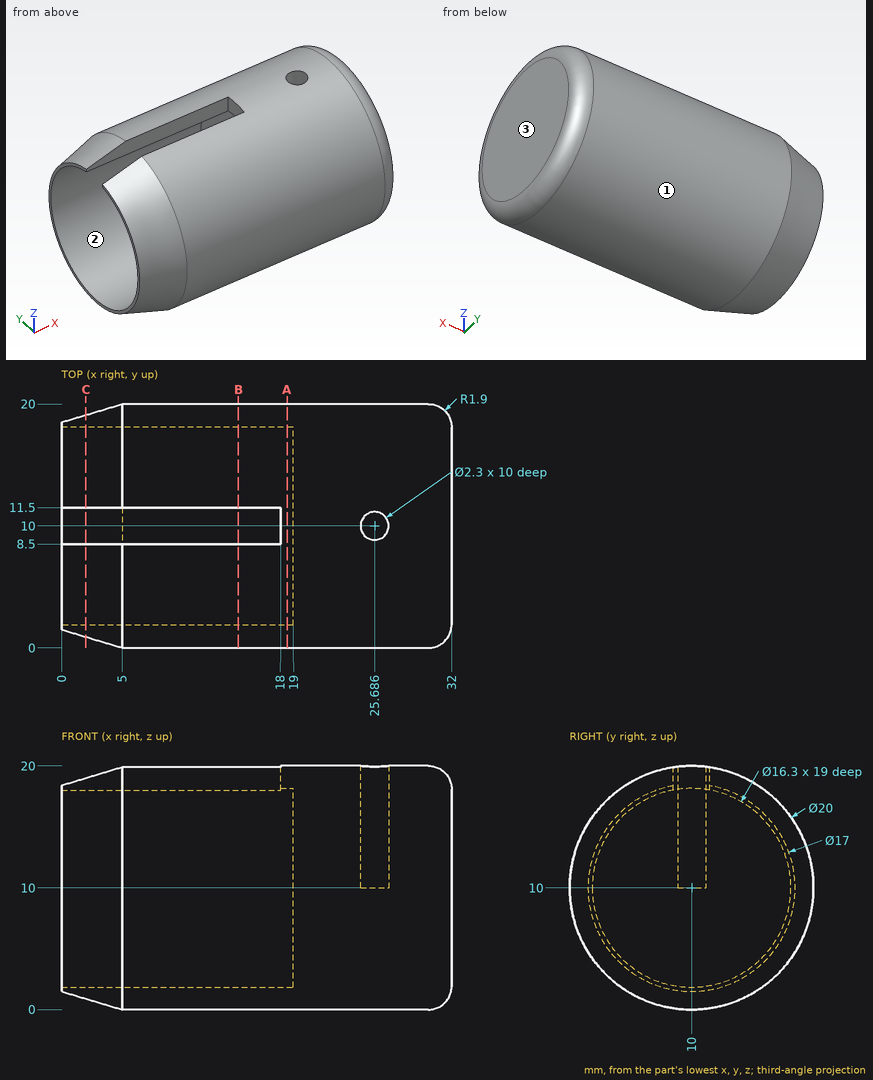
For this review, use the dimensioned drawing (mm, ordinates from the lowest corner) and the shaded views. Give positions to 0.01 mm unless a question says otherwise; leave off trailing zeros. Write each loop counter-clockwise with the first axis right and the second up, starting at its lowest first coordinate (ties: lowest second). Pieces come first, ordered by that corner, then holes.
(1) Consider section B-B, the plane x = 14.5. Give the boundary of the cut face in (y, z).
(2) For P1, Ø1, axis at x = 4.5, z = 16.5, coming from the -Y side; P2, Ø1, axis at x = 25, z = 3.5, coming from the -Y side; P3, Ø4, axis at x = 11, y = 16, coming from the -Z side, all flat-tipped, find the tip position at first contact; note any pin that passes through.
(3) Consider section C-C, the plane x = 2. Give the boundary of the cut face in (y, z), and give its area (3 significant figures).
(4) The part is to be moulded in two halves that separate along Y. For the marked faces 1, 2 and 3, say which applies: released by +Y, released by -Y, zero draft, split by the parting line, or undercut.
(5) To check wall thickness, follow L1, parallel to Y at x = 11, z = 14.75; L2, parallel to Y at x = 4.5, z = 2.5; L3, parallel to X at y = 11.5, z = 10.75. State the ranges of each line that lie inside material, in increasing order.
(6) Consider section A-A, the plane x = 18.5. Give the boundary of the cut face in (y, z).
Returned:
1. outline: (8.5, 18.01) - (8.5, 19.89) arc R10 ccw (long way) to (11.5, 19.89) - (11.5, 18.01) arc R8.15 cw (long way) to start
2. P1: stops at y = 2.14
2. P2: stops at y = 2
2. P3: stops at z = 0.83
3. outline: (8.5, 18.01) - (8.5, 18.98) arc R9.1 ccw (long way) to (11.5, 18.98) - (11.5, 18.01) arc R8.15 cw (long way) to start
3. area: 48.6 mm2
4. face 1: split by the parting line
4. face 2: undercut
4. face 3: zero draft
5. L1: y = 1.2 to 3.38, 16.62 to 18.8
5. L2: y = 3.61 to 6.81, 13.19 to 16.39
5. L3: x = 19 to 32
6. outline: circle Ø20 at (10, 10); hole circle Ø16.3 at (10, 10)
